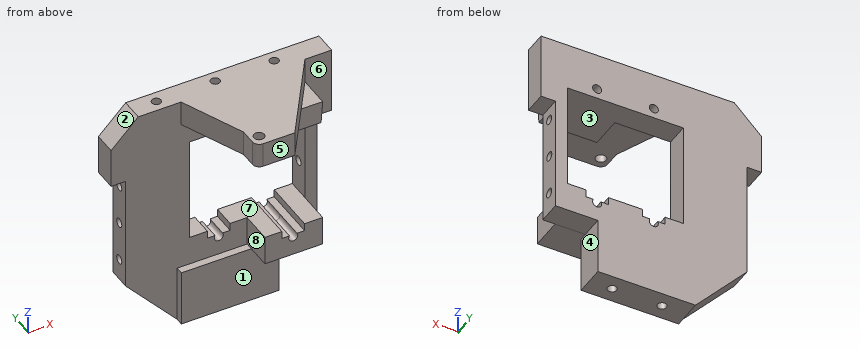
from build123d import *

# Parameters (mm, degrees)
EXTRUDE_1_DEPTH     = 5
SKETCH_4_R          = 0.999999968
SKETCH_4_R_2        = 1.000000188
CUT_EXTRUDE_1_DEPTH = 5
SKETCH_6_R          = 1.000000276
SKETCH_6_R_2        = 0.999999818
CUT_EXTRUDE_2_DEPTH = 5
SKETCH_13_R         = 1.000000021
SKETCH_13_R_2       = 0.999999728
SKETCH_13_R_3       = 0.999999832
CUT_EXTRUDE_3_DEPTH = 6
SKETCH_18_R         = 1.000000534
SKETCH_18_R_2       = 1.000000046
SKETCH_18_R_3       = 0.999998785
CUT_EXTRUDE_5_DEPTH = 3.5
SKETCH_23_R         = 0.999998521
SKETCH_23_R_2       = 0.99999884
SKETCH_23_R_3       = 0.999998599
CUT_EXTRUDE_7_DEPTH = 12
EXTRUDE_5_DEPTH     = 7.05
SKETCH_26_R         = 1.000000188
EXTRUDE_5_2_DEPTH   = 7.05
SKETCH_27_W         = 21.53717804
SKETCH_27_H         = 12.569114685
EXTRUDE_6_DEPTH     = 1.68
SKETCH_28_R         = 1
CUT_EXTRUDE_8_DEPTH = 8
SKETCH_29_R         = 1.149999964
EXTRUDE_7_DEPTH     = 5.530267715


with BuildPart() as part:
    # Sketch 2 → Extrude 1 (new body)
    with BuildSketch(Plane(origin=(0, 0, 0), x_dir=(1, 0, 0), z_dir=(0, 1, 0))):
        Polygon((-16.950000763, 14.201086044), (25.699960709, 14.201086044), (25.699960709, 28.992816925), (22.523960114, 28.992816925), (22.523960114, 54.730998993), (13.161137581, 54.730880737), (13.161137581, 67.299995422), (-8.376040459, 67.299995422), (-19.75, 54.730998993), (-19.75, 28.992816925), (-22.950000763, 28.992816925), (-22.950000763, 20.201086044), align=None)
    extrude(amount=EXTRUDE_1_DEPTH)

    # Sketch 4 → Cut-Extrude 1 (cut)
    with BuildSketch(Plane.XZ):
        with Locations(Location((0.823959914, -22.48135431, 0), (0, 0, 270))):
            Circle(SKETCH_4_R)
        with Locations(Location((13.323959603, -22.481354784, 0), (0, 0, 270))):
            Circle(SKETCH_4_R_2)
        Polygon((-5.676040173, -24.73135376), (19.823959351, -24.73135376), (19.823959351, -48.23135376), (15.823960304, -48.23135376), (15.823960304, -49.931354523), (10.823960304, -49.931354523), (10.823960304, -48.23135376), (3.323960066, -48.23135376), (3.323960066, -49.931354523), (-1.676040053, -49.931354523), (-1.676040053, -48.23135376), (-5.676040173, -48.23135376), align=None)
    extrude(amount=-CUT_EXTRUDE_1_DEPTH, mode=Mode.SUBTRACT)

    # Sketch 6 → Cut-Extrude 2 (cut)
    with BuildSketch(Plane.XZ):
        with Locations((0.823959833, -50.481354106)):
            Circle(SKETCH_6_R)
        with Locations((13.323959879, -50.481354301)):
            Circle(SKETCH_6_R_2)
    extrude(amount=-CUT_EXTRUDE_2_DEPTH, mode=Mode.SUBTRACT)

    # Sketch 13 → Cut-Extrude 3 (cut)
    with BuildSketch(Plane.XY.offset(-14.201086044)):
        with Locations((1.43202298, 2.499998854)):
            Circle(SKETCH_13_R)
        with Locations((14.432022776, 2.500426737)):
            Circle(SKETCH_13_R_2)
        with Locations((-11.56797721, 2.500425343)):
            Circle(SKETCH_13_R_3)
    extrude(amount=-CUT_EXTRUDE_3_DEPTH, mode=Mode.SUBTRACT)

    # Sketch 18 → Cut-Extrude 5 (cut)
    with BuildSketch(Plane(origin=(22.523960114, 0, 0), x_dir=(0, 0, -1), z_dir=(1, 0, 0))):
        with Locations((31.901501235, 2.515246467)):
            Circle(SKETCH_18_R)
        with Locations((40.901397751, 2.558118146)):
            Circle(SKETCH_18_R_2)
        with Locations((49.901297308, 2.515242677)):
            Circle(SKETCH_18_R_3)
    extrude(amount=-CUT_EXTRUDE_5_DEPTH, mode=Mode.SUBTRACT)

    # Sketch 23 → Cut-Extrude 7 (cut)
    with BuildSketch(Plane.ZY.offset(19.75)):
        with Locations((-31.900998993, 2.5)):
            Circle(SKETCH_23_R)
        with Locations((-40.900998993, 2.5)):
            Circle(SKETCH_23_R_2)
        with Locations((-49.900998993, 2.5)):
            Circle(SKETCH_23_R_3)
    extrude(amount=-CUT_EXTRUDE_7_DEPTH, mode=Mode.SUBTRACT)



with BuildPart() as body_2:
    # Sketch 26 → Extrude 5 (new body)
    with BuildSketch(Plane.XZ):
        with BuildLine():
            Line((7.073960185, -48.23135376), (7.073960185, -54.730880737))
            Line((7.073960185, -54.730880737), (19.823959351, -54.730964891))
            Line((19.823959351, -54.730964891), (19.823959351, -48.23135376))
            Line((19.823959351, -48.23135376), (15.823960304, -48.23135376))
            Line((15.823960304, -48.23135376), (15.823960304, -49.931354523))
            Line((15.823960304, -49.931354523), (14.159124462, -49.931354523))
            ThreePointArc((14.159124462, -49.931354523), (13.323959879, -51.481354119), (12.488795296, -49.931354523))
            Line((12.488795296, -49.931354523), (10.823960304, -49.931354523))
            Line((10.823960304, -49.931354523), (10.823960304, -48.23135376))
            Line((10.823960304, -48.23135376), (7.073960185, -48.23135376))
        make_face()
    extrude(amount=EXTRUDE_5_DEPTH)


with BuildPart() as body_3:
    # Sketch 26 → Extrude 5 2 (new body)
    with BuildSketch(Plane.XZ):
        Polygon((6.658313635, -24.73135376), (6.658313635, -19.73135376), (19.823959351, -19.73135376), (19.466256946, -24.73135376), align=None)
        with Locations(Location((13.323959603, -22.481354784, 0), (0, 0, 270))):
            Circle(SKETCH_26_R, mode=Mode.SUBTRACT)
    extrude(amount=EXTRUDE_5_2_DEPTH)


with BuildPart() as part_1:
    add(part.part)

    add(body_2.part)  # Extrude 6 merges body 2
    # Sketch 27 → Extrude 6 (add)
    with BuildSketch(Plane.XZ):
        with Locations((2.392548561, -61.01543808)):
            Rectangle(SKETCH_27_W, SKETCH_27_H)
    extrude(amount=EXTRUDE_6_DEPTH)

    # Sketch 28 → Cut-Extrude 8 (cut)
    with BuildSketch(Plane(origin=(0, 0, -67.299995422), x_dir=(-1, 0, 0), z_dir=(0, 0, -1))):
        with Locations((-8.161137581, 1.66)):
            Circle(SKETCH_28_R)
        with Locations((2.838862419, 1.66)):
            Circle(SKETCH_28_R)
    extrude(amount=-CUT_EXTRUDE_8_DEPTH, mode=Mode.SUBTRACT)


    add(body_3.part)  # Extrude 7 merges body 3
    # Sketch 29 → Extrude 7 (add)
    with BuildSketch(Plane.XY.offset(-19.73135376)):
        with BuildLine():
            Line((-7.494005203, 0), (19.823959351, 0))
            Line((19.823959351, 0), (7.023960114, -18.999999285))
            Line((7.023960114, -18.999999285), (0.005995274, -18.999999285))
            ThreePointArc((0.005995274, -18.999999285), (-1.054664898, -18.560659457), (-1.494004726, -17.499999285))
            Line((-1.494004726, -17.499999285), (-1.494004726, -13.999999523))
            Line((-1.494004726, -13.999999523), (-7.494005203, 0))
        make_face()
        with Locations(Location((0.512218449, -16.535050796, 0), (0, 0, 180))):
            Circle(SKETCH_29_R, mode=Mode.SUBTRACT)
    extrude(amount=EXTRUDE_7_DEPTH)


solid = part_1.part
Model file for the job. Use its own axes, mm. Face numbers are marked on the shaded views. A direction names the side the tool comes from. Round coordinates to 2 decimals unless told otherwise and drop trailing zeros. Loops run counter-clockwise (first coordinate to the right, second up) from the corner with the lowest first, then second, coordinate; pieces in that order, holes last. Notation, with made-up numbers: M -11,-31 L 3,-31 A29 ccw 3,-8 Z; hole C 35,7 d11. An arc over 180 degrees is marked long. One line per question, with ' | ' between items.
1) Band-saw the part on D-D (y = -10). Give the cut face in (x, z), then the cut area to 3 significant figures.
Solved:
outline: M -3.21,-19.73 L 13.09,-19.73 L 13.09,-14.2 L -3.21,-14.2 Z | area: 90.1 mm²
2) Band-saw the part on C-C (x = -13.5). Give the cut face in (y, z), then the cut area to 3 significant figures.
Solved:
outline: M 0,-61.64 L 5,-61.64 L 5,-14.2 L 0,-14.2 Z; hole C 2.5,-49.9 d2; hole C 2.5,-40.9 d2; hole C 2.5,-31.9 d2 | area: 228 mm²
3) Band-saw the part on B-B (x = 10). Give the cut face in (y, z), then the cut area to 3 significant figures.
Solved:
outline: M -14.58,-19.73 L -7.05,-19.73 L -7.05,-24.73 L 5,-24.73 L 5,-14.2 L -14.58,-14.2 Z; M -7.05,-54.73 L -1.68,-54.73 L -1.68,-67.3 L 5,-67.3 L 5,-48.23 L -7.05,-48.23 Z | area: 331 mm²
4) Mould opens along X. For the marked faces 6, 7 and 8 say: +X half, -X half, draft (parallel to the pull), parting line (faces both ways), or undercut.
Solved:
face 6: draft | face 7: undercut | face 8: -X half
5) Flat gauge pins, fed straight in: pin 1 (12 mm diameter, centred on x = 8.5, z = -61, fed in from -Y); pin 2 (1.5 mm diameter, centred on x = 20, y = 3.5, fed in from -Z); pin 3 (4 mm diameter, centred on y = 1.5, z = -40.5, fed in from +X); pin 4 (2 mm diameter, centred on x = 0.51, y = -16.54, fed in from -Z) (3 decimals). Where does each tip first touch, or does it go through?
Solved:
pin 1: stops at y = -1.68 | pin 2: stops at z = -54.73 | pin 3: stops at x = 22.52 | pin 4: passes through
6) 3-axis set-ups, long thin cutter, end or side, ignore diameter. For the marked faces 1, 2, 3, 4 and 5: which of +Z, -Z, +X, -X, +Y, -Y reach the whole face in a straight line?
Solved:
face 1: -Z, +X, -X, -Y | face 2: +Z, -X, +Y, -Y | face 3: +Y, -Y | face 4: -Z, +X, +Y, -Y | face 5: +Z, -Z, +X, -X, -Y
7) Drill centre lines: line 1 along Z through (x, y) = (0, -6.5); line 2 along Y through (x, z) = (-8, -64); line 3 along Y through (x, z) = (-9.5, -48.5). Where is each one in solid material? Low to high.
Solved:
line 1: z = -19.73 to -14.2 | line 2: y = -1.68 to 5 | line 3: y = 0 to 5
8) Band-saw the part on A-A (y = -5.5). Give the cut face in (x, z), then the cut area to 3 significant figures.
Solved:
outline: M -5.14,-19.73 L 6.66,-19.73 L 6.66,-24.73 L 19.47,-24.73 L 19.82,-19.73 L 16.12,-19.73 L 16.12,-14.2 L -5.14,-14.2 Z; M 7.07,-54.73 L 19.82,-54.73 L 19.82,-48.23 L 15.82,-48.23 L 15.82,-49.93 L 14.16,-49.93 A1 cw long 12.49,-49.93 L 10.82,-49.93 L 10.82,-48.23 L 7.07,-48.23 Z; hole C 13.32,-22.48 d2 | area: 251 mm²
